Source: CAD feature listing. Evaluate the final solid. Frame: model axes, mm. A direction names the side the tool comes from. Coordinates: 2 decimals unless noted, no trailing zeros. Write each loop counter-clockwise with the first axis right and the second up, starting at its lowest first coordinate (ties: lowest second). Pieces come first, ordered by that corner, then holes. Notation, with made-up numbers: (39, 16.5) -> (64, 16.5) arc R33 cw to (64, 50.5) -> close; hole circle Ø1 at (-17.5, 63.5). An arc over 180 degrees is marked (long way). One line per item, written item: value. Start each with the question number.
1. First-contact query: P1, Ø2, axis at x = 1.5, z = -16.5, coming from the +Y side; P2, Ø2.5, axis at x = -0.5, y = 5.5, coming from the +Z side; P3, Ø1.8, axis at x = -0.63, y = 4.29, coming from the -Z side. Flat tips, straight axial feed; report the tip coordinate or a pass-through.
2. Mould query, pull axis X, two halves, no side actions, for faces 1 (the flat face through (-10.371, 1, -18)), 2 (the flat face through (9.629, 1, -18)), 3 (the cylindrical face through (0.217, 0.986, -6.826)), 4 (the flat face through (0, 2, -14)). Classes: released by +X, released by -X, zero draft, split by the parting line, or undercut.
3. Section query A-A, the plane x = -0.5. Output: boundary loops of the cut face in (y, z).
4. Line query: line 1 (Z direction, x = 0, y = 0.5); line 2 (Y direction, x = -6.75, z = -17.5); line 3 (Z direction, x = 4.5, y = 3). Output: solid intervals per line, ascending.
5. Section query B-B, the plane z = -21.25. Output: boundary loops of the cut face in (x, y), and give its area (3 significant figures).
6. Access query for faces 5 (the flat face through (0, 3, -25.588)), 6 (the flat face through (0, 6, -23.588)). Directions: +Z, -Z, +X, -X, +Y, -Y. A direction counts if a zero-diameter tool reaches every point of the face in a straight line with its end or side. Return the directions, or none.
7. Section query D-D, the plane y = 2.25. Output: boundary loops of the cut face in (x, z).
8. Section query C-C, the plane x = -8. Output: boundary loops of the cut face in (y, z).
Autodesk Inventor part; units mm, degrees
ref_plane "YZ Plane" through (0, 0, 0) normal (1, 0, 0) x (0, 1, 0)
ref_plane "XZ Plane" through (0, 0, 0) normal (0, 1, 0) x (-1, 0, 0)
ref_plane "XY Plane" through (0, 0, 0) normal (0, 0, 1) x (1, 0, 0)
sketch "Sketch1" plane through (0, 0, 0) normal (0, 1, 0) x (-1, 0, 0)
  line L0 (10.371, -5.5878) -> (-9.629, -5.5878)
  line L1 (-9.629, -5.5878) -> (-9.629, -25.5878)
  line L2 (-9.629, -25.5878) -> (10.371, -25.5878)
  line L3 (10.371, -25.5878) -> (10.371, -5.5878)
  circle A0 centre (0, -7.8026) radius 1
  point P0 (0, 0)
  dimension "d0" = 20
  dimension "d1" = 20
  dimension "d2" = 2
extrude "Extrusion1" add sketch "Sketch1" along normal blind 2
sketch "Sketch2" plane through (0, 2, 0) normal (0, 1, 0) x (1, 0, 0)
  line L0 (9.629, 25.5878) -> (-10.371, 25.5878)
  line L1 (-10.371, 25.5878) -> (9.629, 25.5878)
  line L2 (9.629, 25.5878) -> (9.629, 23.5878)
  line L3 (9.629, 23.5878) -> (-10.371, 23.5878)
  line L4 (-10.371, 23.5878) -> (-10.371, 25.5878)
  point P0 (0, 0)
  dimension "d5" = 20
  dimension "d6" = 2
extrude "Extrusion2" add sketch "Sketch2" along normal blind 5
sketch "Sketch3" plane through (-10.371, 2, -23.5878) normal (0, 0, 1) x (1, 0, 0)
  circle A0 centre (9.7422, 2.2933) radius 1
  point P0 (10.371, -2)
  dimension "d9" = 2
extrude "Extrusion3" cut sketch "Sketch3" against normal blind 5
properties part number "clampforplatform"
Computed values:
1. P1: stops at y = 2
1. P2: stops at z = -23.59
1. P3: passes through
2. face 1: released by -X
2. face 2: released by +X
2. face 3: undercut
2. face 4: zero draft
3. outline: (0, -25.59) -> (3.3, -25.59) -> (3.3, -23.59) -> (2, -23.59) -> (2, -8.67) -> (0, -8.67) -> close; (0, -6.94) -> (2, -6.94) -> (2, -5.59) -> (0, -5.59) -> close; (5.28, -25.59) -> (7, -25.59) -> (7, -23.59) -> (5.28, -23.59) -> close
4. line 1: z = -25.59 to -8.8, -6.8 to -5.59
4. line 2: y = 0 to 2
4. line 3: z = -25.59 to -23.59
5. outline: (-10.37, 0) -> (9.63, 0) -> (9.63, 2) -> (-10.37, 2) -> close
5. area: 40.0 mm²
6. face 5: -Z, +X, -X, +Y, -Y
6. face 6: +Z, +X, -X, +Y
7. outline: (-10.37, -25.59) -> (9.63, -25.59) -> (9.63, -23.59) -> (-10.37, -23.59) -> close
8. outline: (0, -25.59) -> (7, -25.59) -> (7, -23.59) -> (2, -23.59) -> (2, -5.59) -> (0, -5.59) -> close
